Build history of the part. All positions in model axes, mm. Face numbers are marked on the shaded views. A direction names the side the tool comes from. Give positions to 0.01 mm unless a question says otherwise; leave off trailing zeros. Loops run counter-clockwise (first coordinate to the right, second up) from the corner with the lowest first, then second, coordinate; pieces in that order, holes last. Notation, with made-up numbers: M -20.75,15.5 L 29.25,15.5 A24 cw 29.25,46.5 Z; hole C 51.5,-25.75 d5. An arc over 180 degrees is marked long. Answer as a JSON object with one key per item and string values. Group by question number.
1. Slice it at C-C (z = -8.5). List the corners of the cut face in (x, y).
2. Mould opens along X. For the marked faces 1, 2 and 3 say: released by +X, released by -X, zero draft, split by the parting line, or undercut.
3. Slice it at B-B (z = -18.5). List the corners of the cut face in (x, y), then the cut area to 3 significant figures.
4. 3-axis set-ups, long thin cutter, end or side, ignore diameter. For the marked faces 4, 5 and 6: which of +Z, -Z, +X, -X, +Y, -Y reach the whole face in a straight line?
5. Slice it at D-D (x = 27.5). List the corners of the cut face in (y, z), then the cut area to 3 significant figures.
6. Drop flat-ended pins along their axis: pin 1 Ø9.5 at (x, z) = (-40, -21) entering from -Y; pin 2 Ø21.5 at (x, z) = (16.5, 6.5) entering from +Y; pin 3 Ø2 at (x, y) = (7.5, 7) entering from -Z; pin 4 Ø6 at (x, z) = (37.5, -18.5) entering from +Y. Give the stop position or say it passes through.
7. Drill centre lines: line 1 along Z through (x, y) = (-37.5, 14); line 2 along Z through (x, y) = (-37.5, 15.2); line 3 along X through (y, z) = (15.6, -18.5). Where is each one in solid material? Low to high. Write a range as [from, to].
8. Slice it at A-A (x = -37.5). List the corners of the cut face in (y, z).
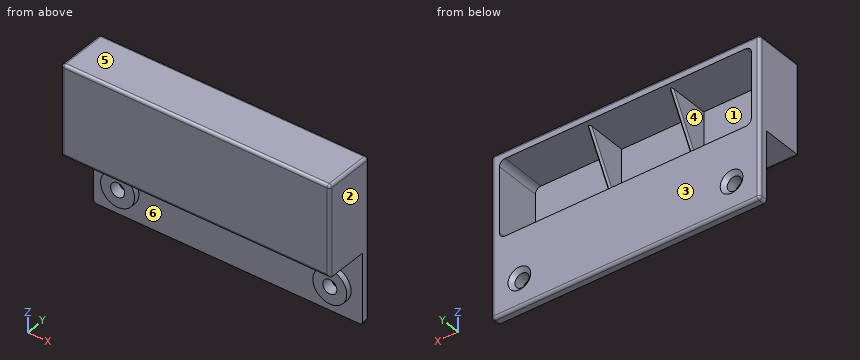
from build123d import *

# Parameters (mm, degrees)
SKETCH2_W                                         = 95
SKETCH2_H                                         = 57
BOSS_EXTRUDE1_DEPTH                               = 18
SKETCH3_W                                         = 25
SKETCH3_H                                         = 15
CUT_EXTRUDE1_DEPTH                                = 101.803025748
CUT_EXTRUDE2_DEPTH                                = 16.5
SKETCH14_R                                        = 6
BOSS_EXTRUDE3_DEPTH                               = 2
CSK_FOR_4_FLAT_HEAD_MACHINE_SCREW_100_D           = 5
CSK_FOR_4_FLAT_HEAD_MACHINE_SCREW_100_CSINK_D     = 8
CSK_FOR_4_FLAT_HEAD_MACHINE_SCREW_100_CSINK_ANGLE = 100
RIB3_START                                        = -0.5
RIB3_DEPTH                                        = 1
RIB11_START                                       = -0.5
RIB11_DEPTH                                       = 1
FILLET1_R                                         = 1
FILLET2_R                                         = 1
FILLET3_R                                         = 1


# Read off the part's stored shape, not the designer's step: Rib3, Rib11
with BuildPart() as part:
    # Sketch2 → Boss-Extrude1 (new body)
    with BuildSketch(Plane(origin=(0, 0, 0), x_dir=(1, 0, 0), z_dir=(0, 1, 0))):
        Rectangle(SKETCH2_W, SKETCH2_H)
    extrude(amount=BOSS_EXTRUDE1_DEPTH)

    # Sketch3 → Cut-Extrude1 (cut, through all)
    with BuildSketch(Plane(origin=(47.5, 0, 0), x_dir=(0, 0, -1), z_dir=(1, 0, 0))):
        with Locations((16, 7.5)):
            Rectangle(SKETCH3_W, SKETCH3_H)
    extrude(amount=-CUT_EXTRUDE1_DEPTH, mode=Mode.SUBTRACT)

    # Sketch4 → Cut-Extrude2 (cut)
    with BuildSketch(Plane(origin=(0, 18, 0), x_dir=(1, 0, 0), z_dir=(0, 1, 0))):
        with BuildLine():
            Line((-42.5, 1.5), (42.5, 1.5))
            ThreePointArc((42.5, 1.5), (43.914213562, 0.914213562), (44.5, -0.5))
            Line((44.5, -0.5), (44.5, -23.5))
            ThreePointArc((44.5, -23.5), (43.914213562, -24.914213562), (42.5, -25.5))
            Line((42.5, -25.5), (-42.5, -25.5))
            ThreePointArc((-42.5, -25.5), (-43.914213562, -24.914213562), (-44.5, -23.5))
            Line((-44.5, -23.5), (-44.5, -0.5))
            ThreePointArc((-44.5, -0.5), (-43.914213562, 0.914213562), (-42.5, 1.5))
        make_face()
    extrude(amount=-CUT_EXTRUDE2_DEPTH, mode=Mode.SUBTRACT)

    # Sketch14 → Boss-Extrude3 (add)
    with BuildSketch(Plane(origin=(0, 15, 0), x_dir=(-1, 0, 0), z_dir=(0, -1, 0))):
        with Locations(Location((37.5, 18.5, 0), (0, 0, 270))):
            Circle(SKETCH14_R)
        with Locations(Location((-37.5, 18.5, 0), (0, 0, 270))):
            Circle(SKETCH14_R)
    extrude(amount=BOSS_EXTRUDE3_DEPTH)

    # CSK for #4 Flat Head Machine Screw (100)3 (through all)
    with Locations(Plane(origin=(37.5, 18, -18.5), x_dir=(0, 0, 1), z_dir=(0, 1, 0))):
        with Locations((0, 0), (0, -75)):
            CounterSinkHole(CSK_FOR_4_FLAT_HEAD_MACHINE_SCREW_100_D / 2, CSK_FOR_4_FLAT_HEAD_MACHINE_SCREW_100_CSINK_D / 2, counter_sink_angle=CSK_FOR_4_FLAT_HEAD_MACHINE_SCREW_100_CSINK_ANGLE)

    # Rib3 outline → Rib3 (add)
    with BuildSketch(Plane.ZY.offset(-14.5).offset(RIB3_START)):
        Polygon((25.5, 16.3125), (-0.833333333, 1.5), (25.5, 1.5), align=None)
    extrude(amount=RIB3_DEPTH)

    # Rib11 outline → Rib11 (add)
    with BuildSketch(Plane(origin=(-14.5, 0, 0), x_dir=(0, 0, -1), z_dir=(1, 0, 0)).offset(RIB11_START)):
        Polygon((0.833333333, 1.5), (-25.5, 16.3125), (-25.5, 1.5), align=None)
    extrude(amount=RIB11_DEPTH)

    # Fillet1
    # the kernel refuses this fillet: 1 mm, written as the material it takes off along each edge
    with BuildSketch(Plane(origin=(-15, 0.274346901, -3.012272176), x_dir=(0, -0.8715755371218976, 0.49026123963727325), z_dir=(0, 0.49026123963727325, 0.8715755371218976))) as fillet1_piece_1_section:
        with BuildLine():
            CenterArc((FILLET1_R, FILLET1_R), FILLET1_R, 180, 90)
            Line((0, FILLET1_R), (0, 0))
            Line((0, 0), (FILLET1_R, 0))
        make_face()
    fillet1_piece_1 = extrude(amount=35.213483756, mode=Mode.PRIVATE)
    fillet1_piece_1 = split(fillet1_piece_1, bisect_by=Plane(origin=(-14.771440182, 8.778475149, 25.5), z_dir=(0, 0, -1)), keep=Keep.TOP, mode=Mode.PRIVATE)
    fillet1_piece_1 = split(fillet1_piece_1, bisect_by=Plane(origin=(-14.771440182, 1.5, 12.560488623), z_dir=(0, 1, 0)), keep=Keep.TOP, mode=Mode.PRIVATE)
    add(fillet1_piece_1, mode=Mode.SUBTRACT)
    with BuildSketch(Plane(origin=(-14, 0.274346901, -3.012272176), x_dir=(-1, 0, 0), z_dir=(0, 0.49026123963727325, 0.8715755371218976))) as fillet1_piece_2_section:
        with BuildLine():
            CenterArc((FILLET1_R, FILLET1_R), FILLET1_R, 180, 90)
            Line((0, FILLET1_R), (0, 0))
            Line((0, 0), (FILLET1_R, 0))
        make_face()
    fillet1_piece_2 = extrude(amount=35.213483756, mode=Mode.PRIVATE)
    fillet1_piece_2 = split(fillet1_piece_2, bisect_by=Plane(origin=(-14.228559818, 8.778475149, 25.5), z_dir=(0, 0, -1)), keep=Keep.TOP, mode=Mode.PRIVATE)
    fillet1_piece_2 = split(fillet1_piece_2, bisect_by=Plane(origin=(-14.228559818, 1.5, 12.560488623), z_dir=(0, 1, 0)), keep=Keep.TOP, mode=Mode.PRIVATE)
    add(fillet1_piece_2, mode=Mode.SUBTRACT)
    with BuildSketch(Plane(origin=(14, 17.538153099, 27.678938843), x_dir=(0, -0.8715755371218977, 0.4902612396372733), z_dir=(0, -0.49026123963727325, -0.8715755371218976))) as fillet1_piece_3_section:
        with BuildLine():
            CenterArc((FILLET1_R, -FILLET1_R), FILLET1_R, 90, 90)
            Line((0, -FILLET1_R), (0, 0))
            Line((0, 0), (FILLET1_R, 0))
        make_face()
    fillet1_piece_3 = extrude(amount=35.213483756, mode=Mode.PRIVATE)
    fillet1_piece_3 = split(fillet1_piece_3, bisect_by=Plane(origin=(14.228559818, 8.778475149, 25.5), z_dir=(0, 0, -1)), keep=Keep.TOP, mode=Mode.PRIVATE)
    fillet1_piece_3 = split(fillet1_piece_3, bisect_by=Plane(origin=(14.228559818, 1.5, 12.560488623), z_dir=(0, 1, 0)), keep=Keep.TOP, mode=Mode.PRIVATE)
    add(fillet1_piece_3, mode=Mode.SUBTRACT)
    with BuildSketch(Plane(origin=(15, 17.538153099, 27.678938843), x_dir=(-1, 0, 0), z_dir=(0, -0.49026123963727325, -0.8715755371218976))) as fillet1_piece_4_section:
        with BuildLine():
            CenterArc((FILLET1_R, -FILLET1_R), FILLET1_R, 90, 90)
            Line((0, -FILLET1_R), (0, 0))
            Line((0, 0), (FILLET1_R, 0))
        make_face()
    fillet1_piece_4 = extrude(amount=35.213483756, mode=Mode.PRIVATE)
    fillet1_piece_4 = split(fillet1_piece_4, bisect_by=Plane(origin=(14.771440182, 8.778475149, 25.5), z_dir=(0, 0, -1)), keep=Keep.TOP, mode=Mode.PRIVATE)
    fillet1_piece_4 = split(fillet1_piece_4, bisect_by=Plane(origin=(14.771440182, 1.5, 12.560488623), z_dir=(0, 1, 0)), keep=Keep.TOP, mode=Mode.PRIVATE)
    add(fillet1_piece_4, mode=Mode.SUBTRACT)

    # Fillet2
    fillet2_edges = [part.edges().sort_by_distance(p)[0] for p in [
        (-47.5, 18, 0),
        (0, 18, 28.5),
        (47.5, 18, 0),
        (0, 0, 28.5),
        (47.5, 9, 28.5),
        (-47.5, 9, 28.5),
        (-47.5, 16.5, -28.5),
        (47.5, 16.5, -28.5),
        (0, 18, -28.5),
    ]]
    fillet(fillet2_edges, radius=FILLET2_R)

    # Fillet3
    # the kernel refuses this fillet: 1 mm, written as the material it takes off along each edge
    with BuildSketch(Plane(origin=(-46.5, 1, 27.5), x_dir=(0, -1, 0), z_dir=(-1, 0, 0))) as fillet3_piece_1_section:
        Polygon((0, 0), (FILLET3_R, 0), (FILLET3_R, FILLET3_R), (0, FILLET3_R), align=None)
    fillet3_piece_1 = extrude(amount=FILLET3_R, mode=Mode.PRIVATE)
    fillet3_piece_1 = fillet3_piece_1 - Plane(origin=(-46.5, 1, 27.5), x_dir=(0, 0.7071067811865475, -0.7071067811865475), z_dir=(-1, 0, 0)) * Sphere(FILLET3_R, mode=Mode.PRIVATE)
    add(fillet3_piece_1, mode=Mode.SUBTRACT)
    with BuildSketch(Plane(origin=(46.5, 1, 27.5), x_dir=(0, -1, 0), z_dir=(1, 0, 0))) as fillet3_piece_2_section:
        Polygon((0, 0), (FILLET3_R, 0), (FILLET3_R, -FILLET3_R), (0, -FILLET3_R), align=None)
    fillet3_piece_2 = extrude(amount=FILLET3_R, mode=Mode.PRIVATE)
    fillet3_piece_2 = fillet3_piece_2 - Plane(origin=(46.5, 1, 27.5), x_dir=(0, 0.7071067811865475, -0.7071067811865475), z_dir=(1, 0, 0)) * Sphere(FILLET3_R, mode=Mode.PRIVATE)
    add(fillet3_piece_2, mode=Mode.SUBTRACT)
    with BuildSketch(Plane(origin=(47.5, 0, -6), x_dir=(0, 1, 0), z_dir=(0, 0, 1)), Plane(origin=(-47.5, 0, 27.5), x_dir=(0, 1, 0), z_dir=(0, 0, -1))) as fillet3_piece_3:
        with BuildLine():
            CenterArc((FILLET3_R, FILLET3_R), FILLET3_R, 180, 90)
            Line((0, FILLET3_R), (0, 0))
            Line((0, 0), (FILLET3_R, 0))
        make_face()
    extrude(amount=33.5, mode=Mode.SUBTRACT)
    with BuildSketch(Plane(origin=(50, 0, -3.5), x_dir=(0, 1, 0), z_dir=(-1, 0, 0))) as fillet3_piece_4:
        with BuildLine():
            CenterArc((FILLET3_R, -FILLET3_R), FILLET3_R, 90, 90)
            Line((0, -FILLET3_R), (0, 0))
            Line((0, 0), (FILLET3_R, 0))
        make_face()
    extrude(amount=100, mode=Mode.SUBTRACT)


solid = part.part
Established:
{
 "1": {"outline": "M -47.5,15 L 47.5,15 L 47.5,17 A1 ccw 46.5,18 L -46.5,18 A1 ccw -47.5,17 Z"},
 "2": {"face 1": "undercut", "face 2": "released by +X", "face 3": "zero draft"},
 "3": {"outline": "M -47.5,15 L -43.5,15 L -43.5,13 L -40,13 L -40,16.74 L -41.5,18 L -46.5,18 A1 ccw -47.5,17 Z; M -35,13 L -31.5,13 L -31.5,15 L 31.5,15 L 31.5,13 L 35,13 L 35,16.74 L 33.5,18 L -33.5,18 L -35,16.74 Z; M 40,13 L 43.5,13 L 43.5,15 L 47.5,15 L 47.5,17 A1 ccw 46.5,18 L 41.5,18 L 40,16.74 Z", "area": "279 mm^2"},
 "4": {"face 4": "+Y", "face 5": "+Z, +X, -X, +Y, -Y", "face 6": "-Y"},
 "5": {"outline": "M 0,-2.5 A1 ccw 1,-3.5 L 15,-3.5 L 15,-28.5 L 17,-28.5 A1 ccw 18,-27.5 L 18,-1.5 L 1.5,-1.5 L 1.5,25.5 L 18,25.5 L 18,27.5 A1 ccw 17,28.5 L 1,28.5 A1 ccw 0,27.5 Z", "area": "205 mm^2"},
 "6": {"pin 1": "stops at y = 13", "pin 2": "stops at y = 18", "pin 3": "stops at z = -3.5", "pin 4": "stops at y = 17.16"},
 "7": {"line 1": "z = [-24.5, -21], [-16, -12.5], [-3.5, -1.5], [25.5, 28.5]", "line 2": "z = [-28.5, -21], [-16, -1.5], [25.5, 28.5]", "line 3": "x = [-47.5, -40], [-35, 35], [40, 47.5]"},
 "8": {"outline": "M 0,-2.5 A1 ccw 1,-3.5 L 15,-3.5 L 15,-12.5 L 13,-12.5 L 13,-16 L 16.74,-16 L 18,-14.5 L 18,-1.5 L 1.5,-1.5 L 1.5,25.5 L 18,25.5 L 18,27.5 A1 ccw 17,28.5 L 1,28.5 A1 ccw 0,27.5 Z; M 13,-24.5 L 15,-24.5 L 15,-28.5 L 17,-28.5 A1 ccw 18,-27.5 L 18,-22.5 L 16.74,-21 L 13,-21 Z"}
}
